Verification items for this drawing (mm, ordinates from the low corner). A direction names the side the tool comes from. Round coordinates to 2 decimals unless told otherwise and drop trailing zeros. Loops run counter-clockwise (first coordinate to the right, second up) from the corner with the lowest first, then second, coordinate; pieces in that order, holes last. Notation, with made-up numbers: (80, 69) - (121, 69) arc R5 cw to (121, 76) - close; hole circle Ø8 at (-25, 59). An arc over 180 degrees is marked (long way). Answer in a Markdown table with one row per item. Add a question column.
(1) Cross-section at C-C on z = 51. Enter the section's corners in (x, y).
(2) Thickness scan on line 1 along Y through (x, z) = (3.15, 4); line 2 along Z through (x, y) = (3.35, 3.25); line 3 along Z through (x, y) = (0.35, 7.75). Record the ranges inside material, lowest first.
(3) Cross-section at B-B on x = 4.4. Enter the section's corners in (y, z).
(4) Access from +Z, -Z, +X, -X, +Y, -Y to the whole of each face (thin tool, end or side, straight path). Record for the marked faces 1 and 2.
(5) Cross-section at D-D on y = 15.5. Enter the section's corners in (x, z), then the cut area to 3 significant figures.
(6) Cross-section at A-A on y = 21.75. Enter the section's corners in (x, z).
(7) Gauge pin test, flat ends, axial feed: pin 1 (2.5 mm diameter, centred on x = 3, z = 2.5, fed in from +Y); pin 2 (2 mm diameter, centred on x = 1, y = 22.5, fed in from -Z); pin 3 (2.5 mm diameter, centred on y = 17, z = 3, fed in from -X). Record the tip position at first contact, or that the pin passes through.
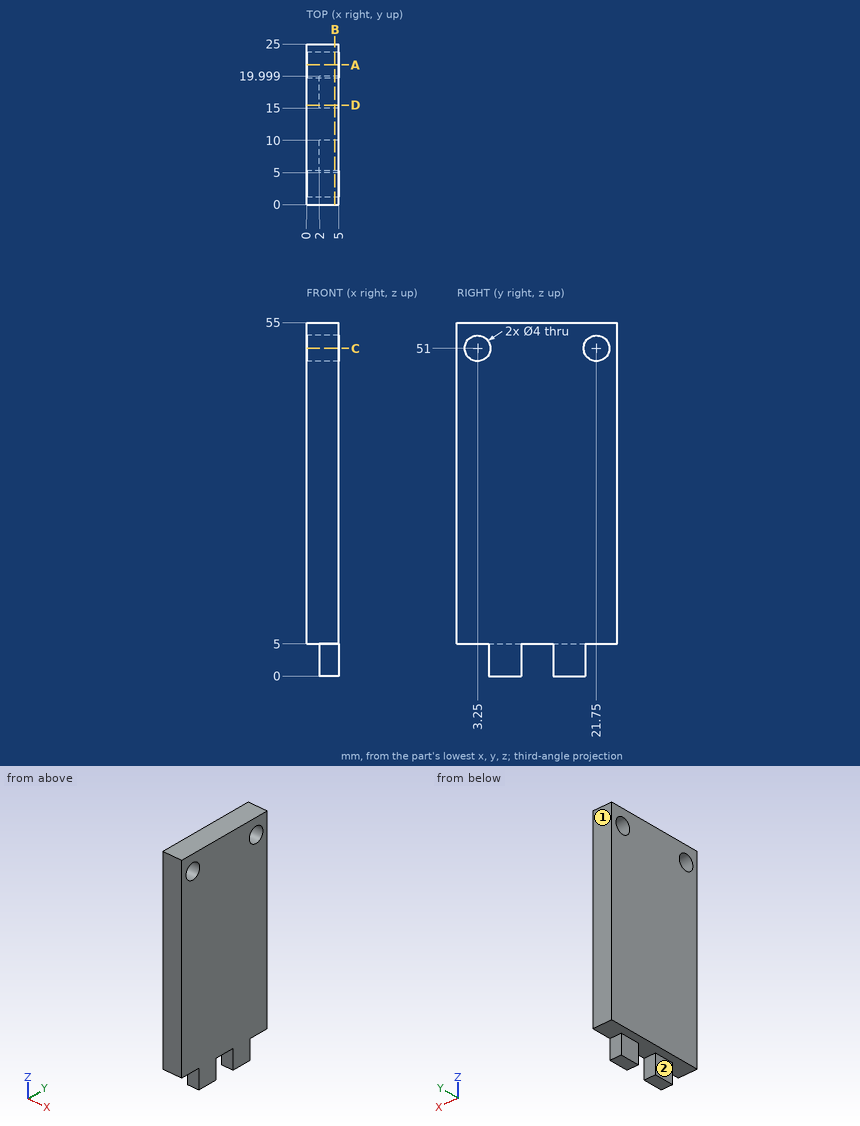
Answers:
| question | item | result |
|---|---|---|
| 1 | outline | (0, 0) - (5, 0) - (5, 1.25) - (0, 1.25) - close; (0, 5.25) - (5, 5.25) - (5, 19.75) - (0, 19.75) - close; (0, 23.75) - (5, 23.75) - (5, 25) - (0, 25) - close |
| 2 | line 1 | y = 5 to 10, 15 to 20 |
| 2 | line 2 | z = 5 to 49, 53 to 55 |
| 2 | line 3 | z = 5 to 55 |
| 3 | outline | (0, 5) - (5, 5) - (5, 0) - (10, 0) - (10, 5) - (15, 5) - (15, 0) - (20, 0) - (20, 5) - (25, 5) - (25, 55) - (0, 55) - close; hole circle Ø4 at (3.25, 51); hole circle Ø4 at (21.75, 51) |
| 4 | face 1 | +Z, -Z, +X, -X, +Y |
| 4 | face 2 | -Z, -X, +Y, -Y |
| 5 | outline | (0, 5) - (2, 5) - (2, 0) - (5, 0) - (5, 55) - (0, 55) - close |
| 5 | area | 265 mm^2 |
| 6 | outline | (0, 5) - (5, 5) - (5, 49) - (0, 49) - close; (0, 53) - (5, 53) - (5, 55) - (0, 55) - close |
| 7 | pin 1 | stops at y = 20 |
| 7 | pin 2 | stops at z = 5 |
| 7 | pin 3 | stops at x = 2 |
